Source: CAD feature listing. Evaluate the final solid. Frame: model axes, mm. A direction names the side the tool comes from. Give positions to 0.01 mm unless a question says otherwise; leave off trailing zeros. Write each loop counter-clockwise with the first axis right and the second up, starting at its lowest first coordinate (ties: lowest second). Pieces come first, ordered by that corner, then holes. Notation, with made-up numbers: (60.25, 75.5) -> (96.25, 75.5) arc R22 ccw to (96.25, 89.5) -> close; hole circle Ø8 at (23.25, 86). An arc over 180 degrees is marked (long way). Write item = value, one per line.
from build123d import *

# Parameters (mm, degrees)
EXTRUDE_3_DEPTH     = 15
CUT_EXTRUDE_1_DEPTH = 30
SHELL_3_T           = -1
EXTRUDE_4_DEPTH     = 12.5
EXTRUDE_4_2_DEPTH   = 12.5
SKETCH_6_R          = 1.6
SKETCH_6_W          = 40
SKETCH_6_H          = 2
EXTRUDE_5_DEPTH     = 3
CUT_EXTRUDE_2_DEPTH = 61


with BuildPart() as part:
    # Sketch 2 → Extrude 3 (new, symmetric)
    with BuildSketch(Plane(origin=(0, 0, 0), x_dir=(0, 0, -1), z_dir=(1, 0, 0))):
        Polygon((-20, 0), (-10, 0), (-32, 12), (-32, 8), align=None)
    extrude(amount=EXTRUDE_3_DEPTH, both=True)

    # Sketch 3 → Cut-Extrude 1 (cut)
    with BuildSketch(Plane(origin=(0, 0, 0), x_dir=(1, 0, 0), z_dir=(0, 1, 0))):
        Polygon((-15, -10), (-15, -32), (-5, -32), align=None)
        Polygon((5, -32), (15, -10), (15, -32), align=None)
    extrude(amount=CUT_EXTRUDE_1_DEPTH, mode=Mode.SUBTRACT)

    # Shell 3
    shell_3_openings = [part.faces().sort_by_distance(p)[0] for p in [
        (0, 10, 32),
        (0, 0, 14.702380952),
    ]]
    offset(amount=SHELL_3_T, openings=shell_3_openings, kind=Kind.INTERSECTION)



with BuildPart() as body_2:
    # Sketch 5 → Extrude 4 (new, symmetric)
    with BuildSketch(Plane.XY):
        Polygon((-19.878151447, 0), (-15.226425738, 12.780511349), (-14.026425738, 12.780511349), (-18.678151447, 0), align=None)
    extrude(amount=EXTRUDE_4_DEPTH, both=True)


with BuildPart() as body_3:
    # Sketch 5 → Extrude 4 2 (new, symmetric)
    with BuildSketch(Plane.XY):
        Polygon((18.678151447, 0), (19.878151447, 0), (15.226425738, 12.780511349), (14.026425738, 12.780511349), align=None)
    extrude(amount=EXTRUDE_4_2_DEPTH, both=True)


with BuildPart() as part_1:
    add(part.part)

    add(body_2.part)  # Extrude 5 merges body 2

    add(body_3.part)  # Extrude 5 merges body 3
    # Sketch 6 → Extrude 5 (add)
    # profile 1 of 3: a face of its own
    with BuildSketch(Plane(origin=(0, 0, 0), x_dir=(1, 0, 0), z_dir=(0, 1, 0))):
        Polygon((-20, -10), (-15, -10), (-10.454545455, -20), (-20, -20), align=None)
        with Locations(Location((-16, -16, 0), (0, 0, 270))):
            Circle(SKETCH_6_R, mode=Mode.SUBTRACT)
    # profile 2 of 3: a face of its own
    with BuildSketch(Plane(origin=(0, 0, 0), x_dir=(1, 0, 0), z_dir=(0, 1, 0))):
        Polygon((20, -20), (20, -10), (15, -10), (10.454545455, -20), align=None)
        with Locations(Location((16, -16, 0), (0, 0, 90))):
            Circle(SKETCH_6_R, mode=Mode.SUBTRACT)
    # profile 3 of 3: a face of its own
    with BuildSketch(Plane(origin=(0, 0, 0), x_dir=(1, 0, 0), z_dir=(0, 1, 0))):
        with Locations((0, 3)):
            Rectangle(SKETCH_6_W, SKETCH_6_H)
    extrude(amount=EXTRUDE_5_DEPTH)

    # Sketch 7 → Cut-Extrude 2 (cut)
    with BuildSketch(Plane(origin=(0, 0, -12.5), x_dir=(-1, 0, 0), z_dir=(0, 0, -1))):
        Polygon((-20, 3), (-18.786240745, 3), (-19.878151447, 0), (-20, 0), align=None)
        Polygon((20, 0), (20, 3), (18.786240745, 3), (19.878151447, 0), align=None)
    extrude(amount=-CUT_EXTRUDE_2_DEPTH, mode=Mode.SUBTRACT)


solid = part_1.part
(1) First-contact query: pin 1 (3 mm diameter, centred on x = 9, y = 7, fed in from +Z); pin 2 (0.6 mm diameter, centred on x = 1, z = -3, fed in from +Y); pin 3 (1 mm diameter, centred on y = 6, z = 27, fed in from -X); pin 4 (8 mm diameter, centred on x = 3.5, z = 4, fed in from +Y). Flat tips, straight axial feed; report the tip coordinate or a pass-through.
Values follow:
pin_1 = 26.5
pin_2 = 3
pin_3 = -7.5
pin_4 = through
(2) Section query B-B (x = -7). Return loops of the section in (y, z).
Values follow:
outline = (0, -4) -> (3, -4) -> (3, -2) -> (0, -2) -> close; (0, 10) -> (9.6, 27.6) -> (5.07, 27.6) -> (0, 20) -> (0, 18.2) -> (4.66, 25.18) -> (7.14, 25.18) -> (0, 12.09) -> close
(3) Section query C-C (y = 2.5). Return loops of the section in (x, z), plus the area to 3 significant figures.
Values follow:
outline = (-18.97, -12.5) -> (-17.77, -12.5) -> (-17.77, -4) -> (17.77, -4) -> (17.77, -12.5) -> (18.97, -12.5) -> (18.97, 20) -> (10.45, 20) -> (8.75, 23.75) -> (-8.75, 23.75) -> (-10.45, 20) -> (-18.97, 20) -> close; hole (-17.77, -2) -> (17.77, -2) -> (17.77, 10) -> (15, 10) -> (12.92, 14.58) -> (-12.92, 14.58) -> (-15, 10) -> (-17.77, 10) -> close; hole circle Ø3.2 at (-16, 16); hole (-10.87, 16.67) -> (10.87, 16.67) -> (8.47, 21.95) -> (-8.47, 21.95) -> close; hole circle Ø3.2 at (16, 16)
area = 330 mm2
(4) Access query for faces 4 (the face through (0, 1, -4)), 5 (the face through (-14.323, 2.146, 11.489)), 6 (the face through (-16, 8, 12.5)), 7 (the face through (0, 1, -2)). Directions: +Z, -Z, +X, -X, +Y, -Y. A direction counts if a zero-diameter tool reaches every point of the face in a straight line with its end or side. Return the directions, or none.
Values follow:
face_4 = -Z, -Y
face_5 = none
face_6 = +Z, +X, -X, +Y
face_7 = -Y
(5) Section query A-A (z = 8). Return loops of the section in (x, y), plus the area to 3 significant figures.
Values follow:
outline = (-19.88, 0) -> (-18.68, 0) -> (-14.03, 12.78) -> (-15.23, 12.78) -> close; (14.03, 12.78) -> (18.68, 0) -> (19.88, 0) -> (15.23, 12.78) -> close
area = 30.7 mm2
(6) Section query D-D (z = 15). Return loops of the section in (x, y), plus the area to 3 significant figures.
Values follow:
outline = (-19.88, 0) -> (-17.25, 0) -> (-17.25, 3) -> (-18.79, 3) -> close; (-14.75, 0) -> (-11.63, 0) -> (-11.63, 1.59) -> (11.63, 1.59) -> (11.63, 0) -> (14.75, 0) -> (14.75, 3) -> (12.73, 3) -> (12.73, 2.73) -> (-12.73, 2.73) -> (-12.73, 3) -> (-14.75, 3) -> close; (17.25, 0) -> (19.88, 0) -> (18.79, 3) -> (17.25, 3) -> close
area = 57.1 mm2
(7) Pull-direction query (Y, two-part tool) for faces 1 (the face through (8.07, 4.6, 22.83)), 2 (the face through (-15, 12.781, 0)), 3 (the face through (15, 1, 20)); classes: pulls with the +Y half, pulls with the -Y half, needs draft (parallel to the pull), parting line crosses it, or undercut.
Values follow:
face_1 = undercut
face_2 = pulls with the +Y half
face_3 = needs draft
(8) Material intervals for line 1 (X direction, y = 0.7, z = 16); line 2 (Z direction, x = 7, y = 1.5); line 3 (X direction, y = 1.65, z = 16), sorted ascending.
Values follow:
line_1 = -19.62 to -17.6, -14.4 to -11.17, 11.17 to 14.4, 17.6 to 19.62
line_2 = -4 to -2, 12.75 to 14.84, 20.45 to 22.25
line_3 = -19.28 to -17.6, -14.4 to -11.17, 11.17 to 14.4, 17.6 to 19.28
